from build123d import *

# Parameters (mm, degrees)
SKETCH_1_R          = 68
SKETCH_1_R_2        = 5.5
EXTRUDE_1_DEPTH     = 60
SKETCH_2_R          = 8.75
CUT_EXTRUDE_1_DEPTH = 10.8
SKETCH_4_R          = 8.75
CUT_EXTRUDE_2_DEPTH = 10.8
CUT_EXTRUDE_START   = -22
SKETCH_6_R          = 68
CUT_EXTRUDE_6_DEPTH = 22
SKETCH_9_R          = 1
CUT_EXTRUDE_7_DEPTH = 104.402127638


with BuildPart() as part:
    # 草图1 → 凸台-拉伸1 (new body)
    with BuildSketch(Plane(origin=(0, 0, 0), x_dir=(1, 0, 0), z_dir=(0, 1, 0))):
        with Locations(Location((0, 0, 0), (0, 0, 270))):
            Circle(SKETCH_1_R)
        with Locations(Location((0, 57, 0), (0, 0, 270))):
            Circle(SKETCH_1_R_2, mode=Mode.SUBTRACT)
        with Locations(Location((28.5, 49.363448016, 0), (0, 0, 270))):
            Circle(SKETCH_1_R_2, mode=Mode.SUBTRACT)
        with Locations(Location((49.363448016, 28.5, 0), (0, 0, 270))):
            Circle(SKETCH_1_R_2, mode=Mode.SUBTRACT)
        with Locations(Location((57, 0, 0), (0, 0, 270))):
            Circle(SKETCH_1_R_2, mode=Mode.SUBTRACT)
        with Locations(Location((49.363448016, -28.5, 0), (0, 0, 270))):
            Circle(SKETCH_1_R_2, mode=Mode.SUBTRACT)
        with Locations(Location((28.5, -49.363448016, 0), (0, 0, 270))):
            Circle(SKETCH_1_R_2, mode=Mode.SUBTRACT)
        with Locations(Location((0, -57, 0), (0, 0, 270))):
            Circle(SKETCH_1_R_2, mode=Mode.SUBTRACT)
        with Locations(Location((-28.5, -49.363448016, 0), (0, 0, 270))):
            Circle(SKETCH_1_R_2, mode=Mode.SUBTRACT)
        with Locations(Location((-49.363448016, -28.5, 0), (0, 0, 270))):
            Circle(SKETCH_1_R_2, mode=Mode.SUBTRACT)
        with Locations(Location((-57, 0, 0), (0, 0, 270))):
            Circle(SKETCH_1_R_2, mode=Mode.SUBTRACT)
        with Locations(Location((-49.363448016, 28.5, 0), (0, 0, 270))):
            Circle(SKETCH_1_R_2, mode=Mode.SUBTRACT)
        with Locations(Location((-28.5, 49.363448016, 0), (0, 0, 270))):
            Circle(SKETCH_1_R_2, mode=Mode.SUBTRACT)
    extrude(amount=EXTRUDE_1_DEPTH)

    # 草图2 → 切除-拉伸1 (cut)
    with BuildSketch(Plane(origin=(0, 60, 0), x_dir=(1, 0, 0), z_dir=(0, 1, 0))):
        with Locations(Location((0, 57, 0), (0, 0, 270))):
            Circle(SKETCH_2_R)
        with Locations(Location((49.363448016, 28.5, 0), (0, 0, 270))):
            Circle(SKETCH_2_R)
        with Locations(Location((49.363448016, -28.5, 0), (0, 0, 270))):
            Circle(SKETCH_2_R)
        with Locations(Location((0, -57, 0), (0, 0, 270))):
            Circle(SKETCH_2_R)
        with Locations(Location((-49.363448016, -28.5, 0), (0, 0, 270))):
            Circle(SKETCH_2_R)
        with Locations(Location((-49.363448016, 28.5, 0), (0, 0, 270))):
            Circle(SKETCH_2_R)
    extrude(amount=-CUT_EXTRUDE_1_DEPTH, mode=Mode.SUBTRACT)

    # 草图4 → 切除-拉伸2 (cut)
    with BuildSketch(Plane.XZ):
        with Locations(Location((28.5, 49.363448016, 0), (0, 0, 270))):
            Circle(SKETCH_4_R)
        with Locations(Location((57, 0, 0), (0, 0, 270))):
            Circle(SKETCH_4_R)
        with Locations(Location((28.5, -49.363448016, 0), (0, 0, 270))):
            Circle(SKETCH_4_R)
        with Locations(Location((-28.5, -49.363448016, 0), (0, 0, 270))):
            Circle(SKETCH_4_R)
        with Locations(Location((-57, 0, 0), (0, 0, 270))):
            Circle(SKETCH_4_R)
        with Locations(Location((-28.5, 49.363448016, 0), (0, 0, 270))):
            Circle(SKETCH_4_R)
    extrude(amount=-CUT_EXTRUDE_2_DEPTH, mode=Mode.SUBTRACT)

    # 草图6 → 切除-拉伸6 (cut)
    with BuildSketch(Plane(origin=(0, 60, 0), x_dir=(1, 0, 0), z_dir=(0, 1, 0)).offset(CUT_EXTRUDE_START)):
        with Locations(Location((0, 0, 0), (0, 0, 270))):
            Circle(SKETCH_6_R)
    extrude(amount=CUT_EXTRUDE_6_DEPTH, mode=Mode.SUBTRACT)

    # 草图8 → 切除-旋转3 (revolve, cut)
    with BuildSketch(Plane.XY):
        with BuildLine():
            Line((0, 38), (0, 0))
            Line((0, 0), (0, -10.414873748))
            ThreePointArc((0, -10.414873748), (48.414873748, 38), (0, 86.414873748))
            Line((0, 86.414873748), (0, 38))
        make_face()
    revolve(axis=Axis((0, -10.414873748, 0), (0, 1, 0)), mode=Mode.SUBTRACT)

    # 草图9 → 切除-拉伸7 (cut, through all)
    with BuildSketch(Plane.XZ):
        with Locations(Location((15.210350017, 58.075311231, 0), (0, 0, 270))):
            Circle(SKETCH_9_R)
        with Locations(Location((42.210205131, 42.689519851, 0), (0, 0, 270))):
            Circle(SKETCH_9_R)
        with Locations(Location((57.899869867, 15.865106101, 0), (0, 0, 270))):
            Circle(SKETCH_9_R)
        with Locations(Location((58.075311231, -15.210350017, 0), (0, 0, 270))):
            Circle(SKETCH_9_R)
        with Locations(Location((42.689519851, -42.210205131, 0), (0, 0, 270))):
            Circle(SKETCH_9_R)
        with Locations(Location((15.865106101, -57.899869867, 0), (0, 0, 270))):
            Circle(SKETCH_9_R)
        with Locations(Location((-15.210350017, -58.075311231, 0), (0, 0, 270))):
            Circle(SKETCH_9_R)
        with Locations(Location((-42.210205131, -42.689519851, 0), (0, 0, 270))):
            Circle(SKETCH_9_R)
        with Locations(Location((-57.899869867, -15.865106101, 0), (0, 0, 270))):
            Circle(SKETCH_9_R)
        with Locations(Location((-58.075311231, 15.210350017, 0), (0, 0, 270))):
            Circle(SKETCH_9_R)
        with Locations(Location((-42.689519851, 42.210205131, 0), (0, 0, 270))):
            Circle(SKETCH_9_R)
        with Locations(Location((-15.865106101, 57.899869867, 0), (0, 0, 270))):
            Circle(SKETCH_9_R)
    extrude(amount=-CUT_EXTRUDE_7_DEPTH, mode=Mode.SUBTRACT)


solid = part.part
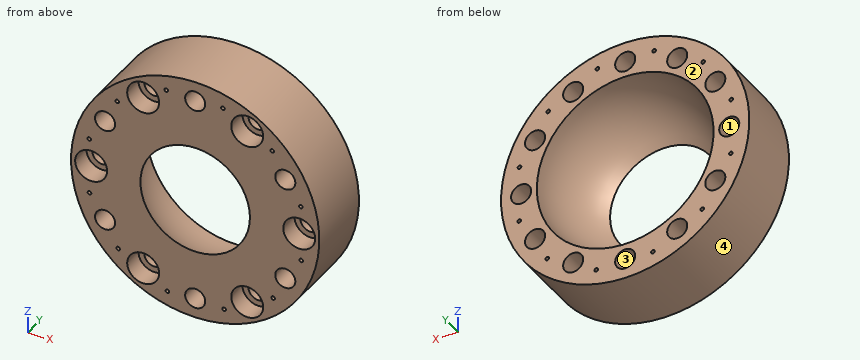
Part model, mm, in its own coordinate system. Face numbers are marked on the shaded views. Give positions to 0.01 mm unless a question says otherwise; leave off trailing zeros. Loops run counter-clockwise (first coordinate to the right, second up) from the corner with the lowest first, then second, coordinate; pieces in that order, holes last.
(1) Drill centre lines: line 1 along Z through (x, y) = (57.5, 18); line 2 along Z through (x, y) = (2, 25.5); line 3 along Z through (x, y) = (57, 19). Where is each one in solid material? Low to high.
Return value:
line 1: z = -36.3 to -16.03, -14.39 to -5.48, 5.48 to 14.95, 16.78 to 36.3
line 2: z = -67.97 to -62.12, -51.88 to -46.73, 46.73 to 51.88, 62.12 to 67.97
line 3: z = -37.08 to -5.5, 5.5 to 15.43, 16.3 to 37.08
(2) Band-saw the part on B-B (x = 0). Write the cut outline in (y, z).
Return value:
outline: (0, -68) - (38, -68) - (38, -62.5) - (0, -62.5) - close; (0, -51.5) - (38, -51.5) - (38, -48.41) arc R48.41 cw to (0, -30) - close; (0, 30) arc R48.41 cw to (38, 48.41) - (38, 51.5) - (0, 51.5) - close; (0, 62.5) - (38, 62.5) - (38, 68) - (0, 68) - close
(3) Band-saw the part on A-A (z = 0). Write the cut outline in (x, y).
Return value:
outline: (-68, 0) - (-65.75, 0) - (-65.75, 10.8) - (-62.5, 10.8) - (-62.5, 38) - (-68, 38) - close; (-51.5, 10.8) - (-48.25, 10.8) - (-48.25, 0) - (-30, 0) arc R48.41 cw to (-48.41, 38) - (-51.5, 38) - close; (30, 0) - (48.25, 0) - (48.25, 10.8) - (51.5, 10.8) - (51.5, 38) - (48.41, 38) arc R48.41 cw to start; (62.5, 10.8) - (65.75, 10.8) - (65.75, 0) - (68, 0) - (68, 38) - (62.5, 38) - close
(4) Pin check, flat tips, straight feed: pin 1 (5 mm diameter, centred on y = 24, z = -47, fed in from +X); pin 2 (5 mm diameter, centred on y = 5.5, z = -13.5, fed in from -X); pin 3 (16 mm diameter, centred on x = -28.5, z = 49.36, fed in from -Y). Stop position of each tip, or through.
Return value:
pin 1: stops at x = 51.42
pin 2: stops at x = -67.1
pin 3: stops at y = 10.8
(5) Band-saw the part on C-C (y = 9). Count the separate pieces of the cut face and the enclosed holes in it, and give its area (3 significant figures).
Return value:
separate pieces: 1
enclosed holes: 25
area: 7,750 mm2
(6) Pull direction X, two halves, no side cores. Call the marked faces 1, 2, 3 and 4: pulls with the +X half, pulls with the -X half, needs draft (parallel to the pull), parting line crosses it, or undercut.
Return value:
face 1: undercut
face 2: needs draft
face 3: undercut
face 4: parting line crosses it
(7) Band-saw the part on D-D (x = -28.5). Write the cut outline in (y, z), and give its area (3 significant figures).
Return value:
outline: (0, -61.74) - (38, -61.74) - (38, -54.86) - (10.8, -54.86) - (10.8, -58.11) - (0, -58.11) - close; (0, -40.61) - (10.8, -40.61) - (10.8, -43.86) - (38, -43.86) - (38, -39.14) arc R39.14 cw to (0, -9.37) - close; (0, 9.37) arc R39.14 cw to (38, 39.14) - (38, 43.86) - (10.8, 43.86) - (10.8, 40.61) - (0, 40.61) - close; (0, 58.11) - (10.8, 58.11) - (10.8, 54.86) - (38, 54.86) - (38, 61.74) - (0, 61.74) - close
area: 1,320 mm2
